Build history of the part. All positions in model axes, mm. A direction names the side the tool comes from. Round coordinates to 2 decimals unless told otherwise and drop trailing zeros. Loops run counter-clockwise (first coordinate to the right, second up) from the corner with the lowest first, then second, coordinate; pieces in that order, holes last. Notation, with made-up numbers: (67, 63) - (116, 63) arc R14 ccw to (116, 79) - close; hole circle Ø1 at (18, 12). An arc over 180 degrees is marked (long way). Put each result on its own line as item: value. Start each with the question number.
from build123d import *

# Parameters (mm, degrees)
F0_W        = 143
F0_H        = 6.35
F2_SIZE     = 0.762
F3_SIZE     = 1.27
F4_R        = 3.175
F5_DEPTH    = 12.7
F6_W        = 15.875
F6_H        = 3.175
F7_DEPTH    = 12.7
F8_R        = 1.5874
F9_T2_ANGLE = 359.64
F9_T4_ANGLE = 359.64


# Not quite as in the source:
# - a fillet or chamfer that OpenCascade refuses, or shapes differently, is made with other operations: its cross-section is extruded or revolved along the edge and cut away or added
# - a fillet or chamfer is up to 0.001 mm smaller than in the source, because OpenCascade refuses the exact size


with BuildPart() as f1:
    # F0 (on Front) → F1 (revolve)
    with BuildSketch(Plane.XZ):
        Polygon((0, 19.05), (-6.35, 19.05), (-6.35, 0), (0, 0), (0, 6.35), align=None)
        with Locations((71.5, 3.175)):
            Rectangle(F0_W, F0_H)
    revolve(axis=Axis((71.5, 0, 0), (1, 0, 0)))

    # F2
    f2_edges = [f1.edges().sort_by_distance(p)[0] for p in [
        (0, 0, -19.05),
        (-6.35, 0, -19.05),
    ]]
    chamfer(f2_edges, length=F2_SIZE)

    # F3
    f3_edges = [f1.edges().sort_by_distance(p)[0] for p in [
        (0, 0, -6.35),
    ]]
    chamfer(f3_edges, length=F3_SIZE)

    # F4 (on Front) → F5 (cut, symmetric)
    with BuildSketch(Plane.XZ):
        with Locations((136, 0)):
            Circle(F4_R)
    extrude(amount=F5_DEPTH, both=True, mode=Mode.SUBTRACT)

    # F6 (on Top) → F7 (cut, symmetric)
    with BuildSketch(Plane.XY):
        with Locations((135.0625, 0)):
            Rectangle(F6_W, F6_H)
    extrude(amount=F7_DEPTH, both=True, mode=Mode.SUBTRACT)

    # F8 (radius 1.5875 in the source; OpenCascade refuses exactly that, so slightly less here)
    f8_edges = [f1.edges().sort_by_distance(p)[0] for p in [
        (127.125, 1.5875, 0),
        (127.125, -1.5875, 0),
    ]]
    fillet(f8_edges, radius=F8_R)

    # F9: fillet of radius 5.08 on 2 edges, made by hand

    # F9_s1 → F9_t2 (revolve, cut)
    with BuildSketch(Plane(origin=(0, 0, 0), x_dir=(1, 0, 0), z_dir=(0, -0.0031415875, 0.9999950652))):
        with BuildLine():
            ThreePointArc((137.92, -6.35), (141.5121024484, -4.8621024484), (143, -1.27))
            Line((143, -1.27), (143, -6.35))
            Line((143, -6.35), (137.92, -6.35))
        make_face()
    revolve(axis=Axis((143, 0, 0), (1, 0, 0)), revolution_arc=F9_T2_ANGLE, mode=Mode.SUBTRACT)

    # F9_s3 → F9_t4 (revolve, cut)
    with BuildSketch(Plane(origin=(0, 0, 0), x_dir=(1, 0, 0), z_dir=(0, 0.0031415875, -0.9999950652))):
        with BuildLine():
            ThreePointArc((137.92, -6.35), (141.5121024484, -4.8621024484), (143, -1.27))
            Line((143, -1.27), (143, -6.35))
            Line((143, -6.35), (137.92, -6.35))
        make_face()
    revolve(axis=Axis((143, 0, 0), (1, 0, 0)), revolution_arc=F9_T4_ANGLE, mode=Mode.SUBTRACT)


solid = f1.part
Item 1: Which spindle directions (+Z, -Z, +X, -X, +Y, -Y) get a long thin tool onto all of the face, cutting with end or side? Do faces 1 (the flat face through (-6.35, 0, 0)), 2 (the cylindrical face through (70.552, -1.907, 6.057)), 3 (the flat face through (132.6, -1.588, 0.1)). Say none if no direction does.
Item 2: Slice it at B-B (x = 96.5). Give the cut face in (y, z).
Item 3: Drill centre lines: probe 1 along X at (y, z) = (-14, -11.5); probe 2 along Z at (x, y) = (136, 4.5) (3 decimals); probe 3 along Z at (x, y) = (87, 0.5). Where is each one in solid material? Low to high. Write a range as [from, to].
Item 4: Drop flat-ended pins along their axis: pin 1 Ø3.5 at (x, z) = (136.5, -1.5) entering from -Y; pin 2 Ø12 at (x, y) = (45.5, -5) entering from -Z; pin 3 Ø18.5 at (y, z) = (-2.5, 8) entering from +X; pin 4 Ø12 at (x, z) = (46.5, -11) entering from -Y. Give the stop position or say it passes through.
Item 5: Two-plate mould, pull along Z, no slides. Class faces 4 (the cylindrical face through (-3.21, 11.59, -15.12)), 5 (the cylindrical face through (138.93, -4, -1.22)), 6 (the flat face through (0, 0, -8)): pulls with the +Z half, pulls with the -Z half, needs draft (parallel to the pull), parting line crosses it, or undercut.
Item 6: Slice it at A-A (x = 136). Give the number of separate pieces and of enclosed holes in the cut face, plus the area to 3 significant figures.
Computed values:
1. face 1: +Z, -Z, -X, +Y, -Y
1. face 2: +X
1. face 3: +Z, -Z, +X
2. outline: circle Ø12.7 at (0, 0)
3. probe 1: x = [-6.35, 0]
3. probe 2: z = [-4.48, -3.175], [3.175, 4.48]
3. probe 3: z = [-6.33, 6.33]
4. pin 1: stops at y = -5.82
4. pin 2: stops at z = -6.35
4. pin 3: stops at x = 142.99
4. pin 4: stops at y = -3.91
5. face 4: parting line crosses it
5. face 5: undercut
5. face 6: needs draft
6. separate pieces: 4
6. enclosed holes: 0
6. area: 29.8 mm^2
